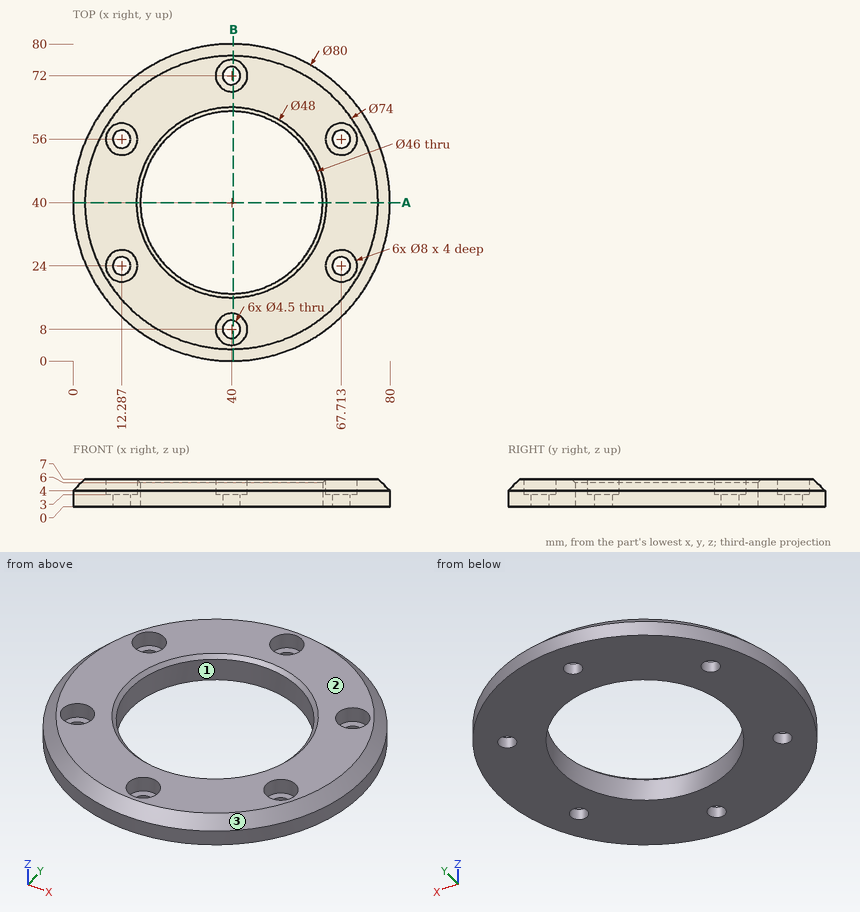
Can you work these out from the drawing? Everything is in mm from the part's minimum corner. Give positions to 0.01 mm unless a question says otherwise; leave off trailing zeros. Write each loop counter-clockwise with the first axis right and the second up, starting at its lowest first coordinate (ties: lowest second). Pieces come first, ordered by that corner, then holes. Notation, with made-up numbers: M 8,1.5 L 51,1.5 A22 ccw 51,22.5 Z; hole C 41.25,-33.75 d8. An arc over 180 degrees is marked long. Answer in a Markdown table with one row per item. Add a question column.
Item 1: For pin 1 Ø4 at (y, z) = (32, 5.5) entering from -X; pin 2 Ø4 at (x, y) = (66.5, 57) entering from +Z; pin 3 Ø4 at (x, y) = (12.29, 24) entering from +Z; pin 4 Ø1 at (x, z) = (55, 2) entering from -Y, each with a flat end and sliding along its axis, tell me the tip position at first contact or that it passes through.
Item 2: Imagine slicing it at B-B, the plane x = 40.5. State how many separate pieces and enclosed holes the cut face has, plus the area to 3 significant figures.
Item 3: Please list where these lines run through material, in increasing order: L1, parallel to Y at x = 42, z = 1.75; L2, parallel to X at y = 72, z = 1.95; L3, parallel to Y at x = 67, z = 4.25 (1 decimal).
Item 4: We'd pull the mould along Y, two halves only. Please class the marked faces 1, 2 and 3: released by +Y, released by -Y, zero draft, split by the parting line, or undercut.
Item 5: Imagine slicing it at A-A, the plane y = 40. Write out the boundary of the cut face in (x, z).
Evaluation:
| question | item | result |
|---|---|---|
| 1 | pin 1 | stops at x = 0.56 |
| 1 | pin 2 | stops at z = 3 |
| 1 | pin 3 | passes through |
| 1 | pin 4 | stops at y = 2.72 |
| 2 | separate pieces | 4 |
| 2 | enclosed holes | 0 |
| 2 | area | 138 mm² |
| 3 | L1 | y = 0.05 to 6.97, 9.03 to 17.09, 62.91 to 70.97, 73.03 to 79.95 |
| 3 | L2 | x = 16 to 37.75, 42.25 to 64 |
| 3 | L3 | y = 10.8 to 20.1, 27.9 to 52.1, 59.9 to 69.2 |
| 4 | face 1 | undercut |
| 4 | face 2 | zero draft |
| 4 | face 3 | split by the parting line |
| 5 | outline | M 0,0 L 17,0 L 17,6 L 16,7 L 3,7 L 0,4 Z; M 63,0 L 80,0 L 80,4 L 77,7 L 64,7 L 63,6 Z |
